from build123d import *

# Parameters (mm, degrees)
F0_W     = 360
F0_H     = 80
F1_DEPTH = 5.5
F2_W     = 360
F2_H     = 5.5
F3_DEPTH = 44.5
F4_R     = 3
F5_DEPTH = 25
F6_R     = 3
F7_DEPTH = 25


with BuildPart() as f1:
    # F0 (on Top) → F1 (new body)
    with BuildSketch(Plane.XY):
        with Locations((180, 40)):
            Rectangle(F0_W, F0_H)
    extrude(amount=F1_DEPTH)

    # F2 (on face) → F3 (join)
    with BuildSketch(Plane(origin=(0, 0, 0), x_dir=(1, 0, 0), z_dir=(0, 0, -1))):
        with Locations((180, -2.75)):
            Rectangle(F2_W, F2_H)
    extrude(amount=F3_DEPTH)

    # F4 (on face) → F5 (cut)
    with BuildSketch(Plane.XZ):
        with Locations((140, -24.5)):
            Circle(F4_R)
        with Locations((240, -24.5)):
            Circle(F4_R)
    extrude(amount=-F5_DEPTH, mode=Mode.SUBTRACT)

    # F6 (on face) → F7 (cut)
    with BuildSketch(Plane(origin=(0, 0, 0), x_dir=(1, 0, 0), z_dir=(0, 0, -1))):
        with Locations((280, -15.5)):
            Circle(F6_R)
        with Locations((280, -55.5)):
            Circle(F6_R)
        with Locations((350, -55.5)):
            Circle(F6_R)
        with Locations((350, -15.5)):
            Circle(F6_R)
    extrude(amount=-F7_DEPTH, mode=Mode.SUBTRACT)


solid = f1.part
Verification items for the finished model (mm, model axes). A direction names the side the tool comes from. Coordinates: 2 decimals unless noted, no trailing zeros. Loops run counter-clockwise (first coordinate to the right, second up) from the corner with the lowest first, then second, coordinate; pieces in that order, holes last. Notation, with made-up numbers: (83.5, 39.25) -> (119.5, 39.25) arc R26 cw to (119.5, 64.25) -> close; hole circle Ø4 at (25.25, 18.5). An arc over 180 degrees is marked (long way). Write each question's results on one line, items separated by ' | '.
Item 1: Mould release check, pull along Y, two halves, no side actions. Record for faces 3 (the face through (277, 15.4, 2.7)), 4 (the face through (177, 0, -19)), 5 (the face through (237, 2.7, -24.4)): +Y half, -Y half, draft (parallel to the pull), parting line (faces both ways), or undercut.
Found:
face 3: undercut | face 4: -Y half | face 5: draft
Item 2: Section check C-C, the plane y = 55.5. Enter the section's corners in (x, z), plus the area to 3 significant figures.
Found:
outline: (0, 0) -> (277, 0) -> (277, 5.5) -> (0, 5.5) -> close; (283, 0) -> (347, 0) -> (347, 5.5) -> (283, 5.5) -> close; (353, 0) -> (360, 0) -> (360, 5.5) -> (353, 5.5) -> close | area: 1,910 mm2
Item 3: Section check B-B, the plane z = -24.5. Enter the section's corners in (x, y), plus the area to 3 significant figures.
Found:
outline: (0, 0) -> (137, 0) -> (137, 5.5) -> (0, 5.5) -> close; (143, 0) -> (237, 0) -> (237, 5.5) -> (143, 5.5) -> close; (243, 0) -> (360, 0) -> (360, 5.5) -> (243, 5.5) -> close | area: 1,910 mm2
Item 4: Section check D-D, the plane x = 280. Enter the section's corners in (y, z), plus the area to 3 significant figures.
Found:
outline: (0, -44.5) -> (5.5, -44.5) -> (5.5, 0) -> (12.5, 0) -> (12.5, 5.5) -> (0, 5.5) -> close; (18.5, 0) -> (52.5, 0) -> (52.5, 5.5) -> (18.5, 5.5) -> close; (58.5, 0) -> (80, 0) -> (80, 5.5) -> (58.5, 5.5) -> close | area: 619 mm2
Item 5: Gauge pin test, flat ends, axial feed: pin 1 (5.5 mm diameter, centred on x = 350, y = 15.5, fed in from -Z); pin 2 (1 mm diameter, centred on x = 273.5, z = -34, fed in from +Y); pin 3 (4 mm diameter, centred on x = 172.5, y = 57.5, fed in from -Z). Record the tip position at first contact, or that the pin passes through.
Found:
pin 1: passes through | pin 2: stops at y = 5.5 | pin 3: stops at z = 0
Item 6: Section check A-A, the plane x = 240. Enter the section's corners in (y, z), plus the area to 3 significant figures.
Found:
outline: (0, -44.5) -> (5.5, -44.5) -> (5.5, -27.5) -> (0, -27.5) -> close; (0, -21.5) -> (5.5, -21.5) -> (5.5, 0) -> (80, 0) -> (80, 5.5) -> (0, 5.5) -> close | area: 652 mm2
Item 7: Material ranges on L1, parallel to Y at x = 280, z = 3.5; L2, parallel to X at y = 3, z = -24; L3, parallel to X at y = 15.5, z = 2.45, recorded low to high.
Found:
L1: y = 0 to 12.5, 18.5 to 52.5, 58.5 to 80 | L2: x = 0 to 137.04, 142.96 to 237.04, 242.96 to 360 | L3: x = 0 to 277, 283 to 347, 353 to 360
Item 8: Tool access check on faces 1 (the face through (177, 43, 0)), 2 (the face through (352.86, 54.6, 2.71)). Record the directions out of +Z, -Z, +X, -X, +Y, -Y that give a thin tool (end or side, any length) a straight path to the whole face; none if there is none.
Found:
face 1: -Z, +X, -X, +Y | face 2: +Z, -Z
